For this review, take the finished solid that the model builds, in its own axes (mm). A direction names the side the tool comes from. Coordinates: 2 decimals unless noted, no trailing zeros. Loops run counter-clockwise (first coordinate to the right, second up) from the corner with the lowest first, then second, coordinate; pieces in that order, holes last. Notation, with made-up numbers: M 17.5,-2 L 22.5,-2 A31 cw 22.5,29 Z; hole C 19,-34 d6. An arc over 180 degrees is marked long. Answer as a JSON object with one key per item and string values. Group by question number.
Item 1: Add section B-B (x = 0). State the section outline as (y, z) points.
Item 2: Mouldability with a two-part tool opening along Y and no side actions: class faces 1 (the face through (0.36, 33.54, -0.88)), 2 (the face through (0, 60, -5)), 3 (the face through (0, 61.1, 0)) as +Y half, -Y half, draft (parallel to the pull), parting line (faces both ways), or undercut.
Item 3: Add section C-C (y = 21.5). State the section outline as (x, z) points, then the cut area to 3 significant figures.
Item 4: Insertion check: pin 1 (10 mm diameter, centred on x = 0.5, y = 25, fed in from -Z); pin 2 (1.4 mm diameter, centred on y = 60.5, z = -2, fed in from +X); pin 3 (1 mm diameter, centred on x = -2.5, y = 60.5, fed in from +Z). Each pin has a flat end and moves straight along its axis. Give the tip position at first contact, or say it passes through.
Item 5: Tool access review of faces 4 (the face through (0, 0, 0)), 5 (the face through (-10, 60, 0)), 6 (the face through (10, 60, 0)), 7 (the face through (-7, 1.6, -4)), 8 (the face through (0, 60, 5)): name each direction out of +Z, -Z, +X, -X, +Y, -Y from which nothing blocks a thin tool from reaching the whole face with its end or side.
Item 6: Wall thickness on L1, parallel to Y at x = -1.75, z = -0.25; L2, parallel to Y at x = -0.25, z = -8.75; L3, parallel to Y at x = -3, z = -3: over which ranges is each line inside the solid? List them lowest first. Write a range as from..to.
Item 7: Add section A-A (z = 0). State the section outline as (x, y) points, then the cut area to 3 significant figures.
from build123d import *

# Parameters (mm, degrees)
RACCORDO2_R                  = 6.4
SCHIZZO5_W                   = 20
SCHIZZO5_H                   = 10
ESTRUSIONE_ESTRUSIONE1_DEPTH = 1.3


with BuildPart() as part:
    # Schizzo4 → Rivoluzione9 (revolve)
    with BuildSketch(Plane.XY, mode=Mode.PRIVATE) as rivoluzione9_sk:
        Polygon((0, 0), (-12.5, 0), (-9.728718708, 1.6), (-0.95, 1.6), (-0.95, 8), (-0.95, 59.8), (0, 59.8), align=None)
    revolve(rivoluzione9_sk.sketch.rotate(Axis((0, -7.357121252, 0), (0, 1, 0)), 270), axis=Axis((0, -7.357121252, 0), (0, 1, 0)))

    # Raccordo2
    raccordo2_edges = [part.edges().sort_by_distance(p)[0] for p in [
        (0, 1.6, 0.95),
    ]]
    fillet(raccordo2_edges, radius=RACCORDO2_R)

    # Schizzo5 → Estrusione-Estrusione1 (add)
    with BuildSketch(Plane(origin=(0, 59.8, 0), x_dir=(1, 0, 0), z_dir=(0, 1, 0))):
        Rectangle(SCHIZZO5_W, SCHIZZO5_H)
    extrude(amount=ESTRUSIONE_ESTRUSIONE1_DEPTH)


solid = part.part
From the geometry:
{
 "1": {"outline": "M 0,-12.5 L 1.6,-9.73 L 1.6,-7.35 A6.4 cw 8,-0.95 L 59.8,-0.95 L 59.8,-5 L 61.1,-5 L 61.1,5 L 59.8,5 L 59.8,0.95 L 8,0.95 A6.4 cw 1.6,7.35 L 1.6,9.73 L 0,12.5 Z"},
 "2": {"face 1": "undercut", "face 2": "draft", "face 3": "+Y half"},
 "3": {"outline": "C 0,0 d1.9", "area": "2.84 mm²"},
 "4": {"pin 1": "stops at z = -0.95", "pin 2": "stops at x = 10", "pin 3": "stops at z = 5"},
 "5": {"face 4": "+Z, -Z, +X, -X, -Y", "face 5": "+Z, -Z, -X, +Y", "face 6": "+Z, -Z, +X, +Y", "face 7": "none", "face 8": "+Z, +X, -X, +Y"},
 "6": {"L1": "y = 0..4.87, 59.8..61.1", "L2": "y = 0..1.6", "L3": "y = 0..2.4, 59.8..61.1"},
 "7": {"outline": "M -12.5,0 L 12.5,0 L 9.73,1.6 L 7.35,1.6 A6.4 cw 0.95,8 L 0.95,59.8 L 10,59.8 L 10,61.1 L -10,61.1 L -10,59.8 L -0.95,59.8 L -0.95,8 A6.4 cw -7.35,1.6 L -9.73,1.6 Z", "area": "190 mm²"}
}
